from build123d import *

# Parameters (mm, degrees)
BOSS_EXTRUDE4_DEPTH = 20
SKETCH12_R          = 1.65
CUT_EXTRUDE1_DEPTH  = 177.068006068
BOSS_EXTRUDE5_DEPTH = 20
CUT_EXTRUDE2_START  = -20
CUT_EXTRUDE2_DEPTH  = 20
LPATTERN2_DEPTH     = 20
CUT_EXTRUDE4_START  = -30
CUT_EXTRUDE4_DEPTH  = 30


with BuildPart() as part:
    # Sketch5 → Boss-Extrude4 (new body)
    with BuildSketch(Plane.XY):
        with BuildLine():
            Line((0, 0), (0, 167.041245738))
            ThreePointArc((0, 167.041245738), (-1.523254023, 168.9835931), (-3.772713274, 167.967252028))
            ThreePointArc((-3.772713274, 167.967252028), (-34.542452011, 86.476422979), (-45, 0))
            Line((-45, 0), (0, 0))
        make_face()
        with BuildLine():
            Line((-1.6, 10), (-39.860221142, 10))
            ThreePointArc((-39.860221142, 10), (-30.000299364, 83.996114978), (-5, 154.335493145))
            ThreePointArc((-5, 154.335493145), (-2.992115624, 155.307611869), (-1.6, 153.56444562))
            Line((-1.6, 153.56444562), (-1.6, 10))
        make_face(mode=Mode.SUBTRACT)
    extrude(amount=BOSS_EXTRUDE4_DEPTH)

    # Sketch12 → Cut-Extrude1 (cut, through all)
    with BuildSketch(Plane.XY.offset(20)):
        with Locations((-40, 5)):
            Circle(SKETCH12_R)
        with Locations((-22.5, 5)):
            Circle(SKETCH12_R)
        with Locations((-5, 5)):
            Circle(SKETCH12_R)
    extrude(amount=-CUT_EXTRUDE1_DEPTH, mode=Mode.SUBTRACT)

    # Sketch14 → Boss-Extrude5 (add)
    with BuildSketch(Plane.XY.offset(20)):
        Polygon((-31.6, 158.56444562), (-1.6, 10), (-3.070322034, 9.703094096), (-33.070322034, 158.267539717), align=None)
    extrude(amount=-BOSS_EXTRUDE5_DEPTH)

    # Sketch17 → Cut-Extrude2 (cut)
    with BuildSketch(Plane.XY.offset(20).offset(CUT_EXTRUDE2_START)):
        Polygon((-120.638203698, 868.825955305), (-109.129206393, -31.174044695), (790.870793607, -19.66504739), (784.13367644, 507.175413991), align=None)
        with BuildLine():
            Line((-45, 0), (0, 0))
            Line((0, 0), (0, 167.041245738))
            ThreePointArc((0, 167.041245738), (-1.523254023, 168.9835931), (-3.772713274, 167.967252028))
            ThreePointArc((-3.772713274, 167.967252028), (-34.542452011, 86.476422979), (-45, 0))
        make_face(mode=Mode.SUBTRACT)
    extrude(amount=CUT_EXTRUDE2_DEPTH, mode=Mode.SUBTRACT)

    # LPattern2: read off the stored shape, not the designer's step
    # LPattern2 outline → LPattern2 (add)
    with BuildSketch(Plane.XY):
        with BuildLine():
            ThreePointArc((-26.929923269, 95.820348103), (-27.373467662, 94.210169532), (-27.809490726, 92.59793799))
            Line((-27.809490726, 92.59793799), (-11.130277006, 10))
            Line((-11.130277006, 10), (-9.6, 10))
            Line((-9.6, 10), (-26.929923269, 95.820348103))
        make_face()
        with BuildLine():
            Line((-17.6, 10), (-31.361118804, 78.147099536))
            ThreePointArc((-31.361118804, 78.147099536), (-31.763386373, 76.327667567), (-32.156172589, 74.506165199))
            Line((-32.156172589, 74.506165199), (-19.130277006, 10))
            Line((-19.130277006, 10), (-17.6, 10))
        make_face()
        with BuildLine():
            Line((-25.6, 10), (-35.278805908, 57.930881129))
            ThreePointArc((-35.278805908, 57.930881129), (-35.62097033, 55.805583127), (-35.950341194, 53.67826488))
            Line((-35.950341194, 53.67826488), (-27.130277006, 10))
            Line((-27.130277006, 10), (-25.6, 10))
        make_face()
        with BuildLine():
            Line((-33.6, 10), (-38.401810118, 33.779275272))
            ThreePointArc((-38.401810118, 33.779275272), (-38.642670237, 31.135229386), (-38.863902948, 28.489468942))
            Line((-38.863902948, 28.489468942), (-35.130277006, 10))
            Line((-35.130277006, 10), (-33.6, 10))
        make_face()
        with BuildLine():
            Line((-39.6, 158.56444562), (-41.070322034, 158.267539717))
            Line((-41.070322034, 158.267539717), (-29.975183074, 103.322767425))
            ThreePointArc((-29.975183074, 103.322767425), (-29.520039112, 104.842464839), (-29.058254032, 106.360157429))
            Line((-29.058254032, 106.360157429), (-39.6, 158.56444562))
        make_face()
        with BuildLine():
            Line((-9.070322034, 158.267539717), (-8.948336076, 157.663447176))
            ThreePointArc((-8.948336076, 157.663447176), (-8.779938618, 158.011942308), (-8.611169445, 158.360257578))
            Line((-8.611169445, 158.360257578), (-9.070322034, 158.267539717))
        make_face()
        with BuildLine():
            Line((-17.070322034, 158.267539717), (-14.508363766, 145.580342723))
            ThreePointArc((-14.508363766, 145.580342723), (-13.985146964, 146.768790335), (-13.457679601, 147.955357539))
            Line((-13.457679601, 147.955357539), (-15.6, 158.56444562))
            Line((-15.6, 158.56444562), (-17.070322034, 158.267539717))
        make_face()
        with BuildLine():
            Line((-25.070322034, 158.267539717), (-19.890886638, 132.618208106))
            ThreePointArc((-19.890886638, 132.618208106), (-19.386082828, 133.896404549), (-18.876440608, 135.172679536))
            Line((-18.876440608, 135.172679536), (-23.6, 158.56444562))
            Line((-23.6, 158.56444562), (-25.070322034, 158.267539717))
        make_face()
        with BuildLine():
            ThreePointArc((-42.198101589, 45.000914697), (-41.903670312, 47.296637828), (-41.594598358, 49.590435769))
            Line((-41.594598358, 49.590435769), (-63.6, 158.56444562))
            Line((-63.6, 158.56444562), (-65.070322034, 158.267539717))
            Line((-65.070322034, 158.267539717), (-42.198101589, 45.000914697))
        make_face()
        with BuildLine():
            ThreePointArc((-38.7019538, 67.304658261), (-38.331864724, 69.236107391), (-37.951310909, 71.165521929))
            Line((-37.951310909, 71.165521929), (-55.6, 158.56444562))
            Line((-55.6, 158.56444562), (-57.070322034, 158.267539717))
            Line((-57.070322034, 158.267539717), (-38.7019538, 67.304658261))
        make_face()
        with BuildLine():
            ThreePointArc((-34.559404558, 86.407326039), (-34.139952511, 88.100097378), (-33.712367751, 89.79083275))
            Line((-33.712367751, 89.79083275), (-47.6, 158.56444562))
            Line((-47.6, 158.56444562), (-49.070322034, 158.267539717))
            Line((-49.070322034, 158.267539717), (-34.559404558, 86.407326039))
        make_face()
        with BuildLine():
            ThreePointArc((-17.043254073, 126.094468165), (-17.541868523, 124.762466617), (-18.035183962, 123.428493465))
            Line((-18.035183962, 123.428493465), (-1.6, 42.039026998))
            Line((-1.6, 42.039026998), (-1.6, 49.617185499))
            Line((-1.6, 49.617185499), (-17.043254073, 126.094468165))
        make_face()
        with BuildLine():
            ThreePointArc((-11.728678792, 139.39308932), (-12.247145872, 138.161094529), (-12.761006653, 136.927171366))
            Line((-12.761006653, 136.927171366), (-1.6, 81.656212497))
            Line((-1.6, 81.656212497), (-1.6, 89.234370998))
            Line((-1.6, 89.234370998), (-11.728678792, 139.39308932))
        make_face()
        with BuildLine():
            ThreePointArc((-6.2238307, 151.749451318), (-6.759005375, 150.601509463), (-7.290112892, 149.451680241))
            Line((-7.290112892, 149.451680241), (-1.6, 121.273397996))
            Line((-1.6, 121.273397996), (-1.6, 128.851556496))
            Line((-1.6, 128.851556496), (-6.2238307, 151.749451318))
        make_face()
        Polygon((0, 41.693748399), (0, 34.115589899), (4.929677966, 9.703094096), (6.4, 10), align=None)
        Polygon((0, 158.483672593), (0, 152.967146395), (28.929677966, 9.703094096), (30.4, 10), (0.4, 158.56444562), align=None)
        Polygon((0, 120.928119397), (0, 113.349960896), (20.929677966, 9.703094096), (22.4, 10), align=None)
        Polygon((0, 81.310933898), (0, 73.732775397), (12.929677966, 9.703094096), (14.4, 10), align=None)
    extrude(amount=LPATTERN2_DEPTH)

    # Sketch19 → Cut-Extrude4 (cut)
    with BuildSketch(Plane.XY.offset(20).offset(CUT_EXTRUDE4_START)):
        Polygon((-113.909990018, -19.131609845), (183.246695872, -29.17634289), (134.697152825, 220.267861041), (-171.248674479, 235.334960607), align=None)
        with BuildLine():
            Line((-45, 0), (0, 0))
            Line((0, 0), (0, 167.041245738))
            ThreePointArc((0, 167.041245738), (-1.523254023, 168.9835931), (-3.772713274, 167.967252028))
            ThreePointArc((-3.772713274, 167.967252028), (-34.542452011, 86.476422979), (-45, 0))
        make_face(mode=Mode.SUBTRACT)
    extrude(amount=CUT_EXTRUDE4_DEPTH, mode=Mode.SUBTRACT)


solid = part.part
The listing builds one solid part. Answer for the finished solid, in the listing's coordinates (mm). A direction names the side the tool comes from. Give positions to 0.01 mm unless a question says otherwise; leave off trailing zeros. Order: outer loops, then holes, each group sorted by start corner. A loop starts at its lowest first (then second) coordinate and runs counter-clockwise, first axis right, second up. Notation, with made-up numbers: (42.25, 46) - (53.25, 46) arc R22 cw to (53.25, 78) - close; hole circle Ø8 at (15.5, -32.5). An arc over 180 degrees is marked (long way). Answer as CSV lines item,"result".
Q1. A cutting plane is placed at C-C, the plane z = 18.25. Count the separate pieces of the cut face and the enclosed holes in it, and give its area (3 significant figures).
Answer key:
separate pieces,"1"
enclosed holes,"12"
area,"2,230 mm^2"
Q2. Determine the mould class of faces 3 (the face through (-34.25, 87.66, 9.86)), 4 (the face through (-14, 66, 20)), 5 (the face through (-24.384, 43.597, 9.86)) for opening direction Y: pulls with the +Y half, pulls with the -Y half, needs draft (parallel to the pull), parting line crosses it, or undercut.
Answer key:
face 3,"pulls with the +Y half"
face 4,"needs draft"
face 5,"undercut"
Q3. Straight lines are drawn through the part: L1, parallel to X at y = 31.5, z = 15; L2, parallel to X at y = 130, z = 8; L3, parallel to X at y = 107, z = 15. For each, find the intervals that lie inside material, in ascending order.
Answer key:
L1,"x = -43.63 to -37.94, -31.47 to -29.94, -23.47 to -21.94, -15.47 to -13.94, -7.47 to -5.94, -1.6 to 0"
L2,"x = -20.91 to -15.55, -11.36 to -9.83, -3.36 to -1.83, -1.6 to 0"
L3,"x = -28.86 to -23.63, -22.72 to -21.19, -14.72 to -13.19, -6.72 to -5.19, -1.6 to 0"
Q4. A cutting plane is placed at A-A, the plane y = 5. Determine the outline of the cut face in (x, z).
Answer key:
outline,"(-44.97, 0) - (-41.65, 0) - (-41.65, 20) - (-44.97, 20) - close; (-38.35, 0) - (-24.15, 0) - (-24.15, 20) - (-38.35, 20) - close; (-20.85, 0) - (-6.65, 0) - (-6.65, 20) - (-20.85, 20) - close; (-3.35, 0) - (0, 0) - (0, 20) - (-3.35, 20) - close"
Q5. A cutting plane is placed at B-B, the plane y = 51.5. Determine the outline of the cut face in (x, z).
Answer key:
outline,"(-41.33, 0) - (-36.27, 0) - (-36.27, 20) - (-41.33, 20) - close; (-35.51, 0) - (-33.98, 0) - (-33.98, 20) - (-35.51, 20) - close; (-27.51, 0) - (-25.98, 0) - (-25.98, 20) - (-27.51, 20) - close; (-19.51, 0) - (-17.98, 0) - (-17.98, 20) - (-19.51, 20) - close; (-11.51, 0) - (-9.98, 0) - (-9.98, 20) - (-11.51, 20) - close; (-3.51, 0) - (-1.98, 0) - (-1.98, 20) - (-3.51, 20) - close; (-1.6, 0) - (0, 0) - (0, 20) - (-1.6, 20) - close"
Q6. Each of these flat-tipped pins is pushed along its axis until it touches: pin 1 Ø6 at (y, z) = (25.5, 10.5) entering from -X; pin 2 Ø10 at (y, z) = (144.5, 7) entering from -X; pin 3 Ø3 at (x, z) = (-6.5, 5) entering from +Y. Where does it stop, or does it pass through?
Answer key:
pin 1,"stops at x = -44.3"
pin 2,"stops at x = -17.11"
pin 3,"stops at y = 165.6"
Q7. Which of the six approach directions +Z, -Z, +X, -X, +Y, -Y give full straight-line access (tool end or side, diameter ignored) to faces 1 (the face through (-23, 0, 10)), 2 (the face through (-19.587, 51.877, 9.86))?
Answer key:
face 1,"+Z, -Z, +X, -X, -Y"
face 2,"+Z, -Z"
Q8. A cutting plane is placed at D-D, the plane y = 131. Determine the outline of the cut face in (x, z).
Answer key:
outline,"(-20.52, 0) - (-15.15, 0) - (-15.15, 20) - (-20.52, 20) - close; (-11.56, 0) - (-10.03, 0) - (-10.03, 20) - (-11.56, 20) - close; (-3.56, 0) - (-2.03, 0) - (-2.03, 20) - (-3.56, 20) - close; (-1.6, 0) - (0, 0) - (0, 20) - (-1.6, 20) - close"
